Design review of the part built by this model. Coordinates are the model's own, in mm. A direction names the side the tool comes from. Coordinates: 2 decimals unless noted, no trailing zeros. Write each loop counter-clockwise with the first axis right and the second up, starting at its lowest first coordinate (ties: lowest second). Pieces come first, ordered by that corner, then holes. Notation, with made-up numbers: (-14.5, -16.75) -> (32.5, -16.75) arc R28 ccw to (32.5, 19.25) -> close; hole circle Ø9 at (85.25, 64). An arc over 180 degrees is marked (long way). One line per question, with ' | ' between items. Start each with the question number.
Q1. Add section B-B on y = 0. State the section outline as (x, z) points, and give its area (3 significant figures).
Q2. Wall thickness on probe 1 along Y at (x, z) = (-24.5, 8.75); probe 2 along X at (y, z) = (7, 3); probe 3 along Y at (x, z) = (21, 0.5): over which ranges is each line inside the solid? List them lowest first.
Q3. Add section D-D on y = -15. State the section outline as (x, z) points.
Q4. Add section A-A on z = 7.5. State the section outline as (x, y) points.
Q5. Add section C-C on x = 18.5. State the section outline as (y, z) points, and give its area (3 significant figures).
Q6. For P1, Ø0.8, axis at x = 41.5, y = 21.5, coming from the +Z side; P2, Ø0.8, axis at x = 42, y = 21.5, coming from the -Z side; P3, Ø0.8, axis at x = 41.5, z = 3.5, coming from the -Y side, all flat-tipped, find the tip position at first contact; note any pin that passes through.
Q7. For faces 1 (the flat face through (-1, 0, 6.3)), 2 (the flat face through (42.5, -22, 3)), list the 3-axis set-ups (+Z, -Z, +X, -X, +Y, -Y) from which the entire face can be reached by the end or side of a thin tool; tool diameter is ignored.
from build123d import *

# Parameters (mm, degrees)
F0_W     = 82
F0_H     = 54
F1_DEPTH = 9.5
F2_W     = 82
F2_H     = 2
F3_DEPTH = 3.2
F4_W     = 3.5
F4_H     = 4.8
F6_DEPTH = 1.5
F5_W     = 3.5
F5_H     = 4.8
F7_DEPTH = 1.5


with BuildPart() as f1:
    # F0 (on Top) → F1 (new body)
    with BuildSketch(Plane.XY):
        Rectangle(F0_W, F0_H)
    extrude(amount=F1_DEPTH)

    # F2 (on face) → F3 (cut)
    with BuildSketch(Plane.XY.offset(9.5)):
        Rectangle(F2_W, F2_H)
    extrude(amount=-F3_DEPTH, mode=Mode.SUBTRACT)

    # F4 (on face) → F6 (join)
    with BuildSketch(Plane.XZ.offset(27)):
        with Locations((27.75, 3.4)):
            Rectangle(F4_W, F4_H)
        with Locations((-27.25, 3.4)):
            Rectangle(F4_W, F4_H)
    extrude(amount=F6_DEPTH)

    # F5 (on face) → F7 (join)
    with BuildSketch(Plane.YZ.offset(41)):
        with Locations((-22.25, 3.4)):
            Rectangle(F5_W, F5_H)
        with Locations((0, 3.4)):
            Rectangle(F5_W, F5_H)
        with Locations((22.25, 3.4)):
            Rectangle(F5_W, F5_H)
    extrude(amount=F7_DEPTH)


solid = f1.part
Output values:
1) outline: (-41, 0) -> (41, 0) -> (41, 1) -> (42.5, 1) -> (42.5, 5.8) -> (41, 5.8) -> (41, 6.3) -> (-41, 6.3) -> close | area: 524 mm2
2) probe 1: y = -27 to -1, 1 to 27 | probe 2: x = -41 to 41 | probe 3: y = -27 to 27
3) outline: (-41, 0) -> (41, 0) -> (41, 9.5) -> (-41, 9.5) -> close
4) outline: (-41, -27) -> (41, -27) -> (41, -1) -> (-41, -1) -> close; (-41, 1) -> (41, 1) -> (41, 27) -> (-41, 27) -> close
5) outline: (-27, 0) -> (27, 0) -> (27, 9.5) -> (1, 9.5) -> (1, 6.3) -> (-1, 6.3) -> (-1, 9.5) -> (-27, 9.5) -> close | area: 507 mm2
6) P1: stops at z = 5.8 | P2: stops at z = 1 | P3: stops at y = -24
7) face 1: +Z, +X, -X | face 2: +Z, -Z, +X, +Y, -Y
